```python
from build123d import *

# Parameters (mm, degrees)
F1_DEPTH = 19.05
F2_R     = 4.445
F3_DEPTH = 25.4
F4_R     = 4.445
F5_DEPTH = 3.175
F6_R     = 1.5875
F7_SIZE  = 0.762


with BuildPart() as f1:
    # F0 (on Right) → F1 (new body)
    with BuildSketch(Plane.YZ):
        Polygon((0, 3.175), (0, 0), (26.542, 0), (26.542, 32.258), (0, 32.258), (0, 29.083), (23.367, 29.083), (23.367, 3.175), align=None)
    extrude(amount=F1_DEPTH)

    # F2 (on face) → F3 (cut)
    with BuildSketch(Plane.XY.offset(3.175)):
        with Locations((9.525, 7.62)):
            Circle(F2_R)
    extrude(amount=-F3_DEPTH, mode=Mode.SUBTRACT)

    # F4 (on face) → F5 (cut, through all)
    with BuildSketch(Plane.XY.offset(32.258)):
        with Locations((9.525, 7.62)):
            Circle(F4_R)
    extrude(amount=-F5_DEPTH, mode=Mode.SUBTRACT)

    # F6
    f6_edges = [f1.edges().sort_by_distance(p)[0] for p in [
        (19.05, 0, 30.6705),
        (0, 0, 30.6705),
        (0, 0, 1.5875),
        (19.05, 0, 1.5875),
        (9.525, 26.542, 32.258),
        (9.525, 26.542, 0),
    ]]
    fillet(f6_edges, radius=F6_R)

    # F7
    f7_edges = [f1.edges().sort_by_distance(p)[0] for p in [
        (5.08, 7.62, 0),
        (5.08, 7.62, 29.083),
        (5.08, 7.62, 32.258),
        (5.08, 7.62, 3.175),
    ]]
    chamfer(f7_edges, length=F7_SIZE)


solid = f1.part
```
Read the model definition and answer for the solid it produces. Units are mm, in the model's axes. Give positions to 0.01 mm unless a question says otherwise; leave off trailing zeros. Write each loop counter-clockwise with the first axis right and the second up, starting at its lowest first coordinate (ties: lowest second). Pieces come first, ordered by that corner, then holes. Notation, with made-up numbers: (49.25, -38.5) - (61.25, -38.5) arc R25 cw to (61.25, -8.5) - close; hole circle Ø4 at (89.5, 7). An arc over 180 degrees is marked (long way). Write item = value, one per line. Start each with the question number.
Item 1: The mould has two halves that part along Z. Classify faces 1 (the cylindrical face through (9.66, 26.06, 0.45)), 2 (the flat face through (9, 23.367, 16)), 3 (the flat face through (19.05, 24, 15)), 4 (the flat face through (9, 14, 3.175)): +Z half, -Z half, draft (parallel to the pull), parting line (faces both ways), or undercut.
Item 2: Find section C-C (x = 16). Give the vertices of the cut face in (y, z) (1 decimal).
Item 3: Find section B-B (y = 19.5). Give the vertices of the cut face in (x, z) (3 decimals).
Item 4: Find section D-D (z = 13). Give the vertices of the cut face in (x, y), then the cut area to 3 significant figures.
Item 5: Find the intervals of material crossed by probe 1 along Z at (x, y) = (12.5, 15.5) (3 decimals); probe 2 along Y at (x, z) = (16.25, 12); probe 3 along Z at (x, y) = (4.75, 9.5), in increasing order. Write a range as [from, to].
Item 6: This flat-tipped pin is pushed along its axis until it touches: P1, Ø5.5, axis at x = 5.5, z = 13.5, coming from the -Y side. Where does it stop, or does it pass through?
Item 7: Find section A-A (y = 7.62). Give the vertices of the cut face in (x, z) (3 decimals).
Response:
q1.face_1 = -Z half
q1.face_2 = undercut
q1.face_3 = draft
q1.face_4 = undercut
q2.outline = (0, 0) - (25, 0) arc R1.6 ccw to (26.5, 1.6) - (26.5, 30.7) arc R1.6 ccw to (25, 32.3) - (0, 32.3) - (0, 29.1) - (23.4, 29.1) - (23.4, 3.2) - (0, 3.2) - close
q3.outline = (0, 0) - (19.05, 0) - (19.05, 3.175) - (0, 3.175) - close; (0, 29.083) - (19.05, 29.083) - (19.05, 32.258) - (0, 32.258) - close
q4.outline = (0, 23.37) - (19.05, 23.37) - (19.05, 26.54) - (0, 26.54) - close
q4.area = 60.5 mm²
q5.probe_1 = [0, 3.175], [29.083, 32.258]
q5.probe_2 = [23.37, 26.54]
q5.probe_3 = [0.08, 3.1], [29.16, 32.18]
q6.P1 = 23.37
q7.outline = (0, 0) - (4.318, 0) - (5.08, 0.762) - (5.08, 2.413) - (4.318, 3.175) - (0, 3.175) - close; (0, 29.083) - (4.318, 29.083) - (5.08, 29.845) - (5.08, 31.496) - (4.318, 32.258) - (0, 32.258) - close; (13.97, 0.762) - (14.732, 0) - (19.05, 0) - (19.05, 3.175) - (14.732, 3.175) - (13.97, 2.413) - close; (13.97, 29.845) - (14.732, 29.083) - (19.05, 29.083) - (19.05, 32.258) - (14.732, 32.258) - (13.97, 31.496) - close
